from build123d import *

# Parameters (mm, degrees)
SKETCH_1_R      = 27
EXTRUDE_1_DEPTH = 47


with BuildPart() as part:
    # Эскиз1 → Бобышка-Вытянуть1 (new body)
    with BuildSketch(Plane(origin=(0, 0, 0), x_dir=(1, 0, 0), z_dir=(0, 1, 0))):
        with BuildLine():
            ThreePointArc((47, 0), (33.234018716, 33.234018716), (0, 47))
            ThreePointArc((0, 47), (-33.234018716, 33.234018716), (-47, 0))
            ThreePointArc((-47, 0), (-33.234018716, -33.234018716), (0, -47))
            ThreePointArc((0, -47), (33.234018716, -33.234018716), (47, 0))
        make_face()
        Circle(SKETCH_1_R, mode=Mode.SUBTRACT)
        with BuildLine():
            ThreePointArc((-47, 0), (-43.422338028, 17.986121321), (-33.234018716, 33.234018716))
            Line((-33.234018716, 33.234018716), (-56.922095886, 56.922095886))
            ThreePointArc((-56.922095886, 56.922095886), (-57.279535343, 27.533981904), (-47, 0))
        make_face()
        with BuildLine():
            ThreePointArc((-33.234018716, 33.234018716), (-17.986121321, 43.422338028), (0, 47))
            Line((0, 47), (0, 80.5))
            ThreePointArc((0, 80.5), (-21.033282547, 59.972213182), (-33.234018716, 33.234018716))
        make_face()
        with BuildLine():
            Line((33.234018716, 33.234018716), (56.922095886, 56.922095886))
            ThreePointArc((56.922095886, 56.922095886), (27.533981904, 57.279535343), (0, 47))
            ThreePointArc((0, 47), (17.986121321, 43.422338028), (33.234018716, 33.234018716))
        make_face()
        with BuildLine():
            ThreePointArc((80.5, 0), (59.972213182, 21.033282547), (33.234018716, 33.234018716))
            ThreePointArc((33.234018716, 33.234018716), (43.422338028, 17.986121321), (47, 0))
            Line((47, 0), (80.5, 0))
        make_face()
        with BuildLine():
            ThreePointArc((56.922095886, -56.922095886), (57.279535343, -27.533981904), (47, 0))
            ThreePointArc((47, 0), (43.422338028, -17.986121321), (33.234018716, -33.234018716))
            Line((33.234018716, -33.234018716), (56.922095886, -56.922095886))
        make_face()
        with BuildLine():
            ThreePointArc((0, -80.5), (21.033282547, -59.972213182), (33.234018716, -33.234018716))
            ThreePointArc((33.234018716, -33.234018716), (17.986121321, -43.422338028), (0, -47))
            Line((0, -47), (0, -80.5))
        make_face()
        with BuildLine():
            ThreePointArc((-56.922095886, -56.922095886), (-27.533981904, -57.279535343), (0, -47))
            ThreePointArc((0, -47), (-17.986121321, -43.422338028), (-33.234018716, -33.234018716))
            Line((-33.234018716, -33.234018716), (-56.922095886, -56.922095886))
        make_face()
        with BuildLine():
            ThreePointArc((-33.234018716, -33.234018716), (-43.422338028, -17.986121321), (-47, 0))
            Line((-47, 0), (-80.5, 0))
            ThreePointArc((-80.5, 0), (-59.972213182, -21.033282547), (-33.234018716, -33.234018716))
        make_face()
    extrude(amount=EXTRUDE_1_DEPTH)


solid = part.part
Read the model definition and answer for the solid it produces. Units are mm, in the model's axes. A direction names the side the tool comes from. Round coordinates to 2 decimals unless told otherwise and drop trailing zeros. Order: outer loops, then holes, each group sorted by start corner. A loop starts at its lowest first (then second) coordinate and runs counter-clockwise, first axis right, second up.
1) The part is cut by section A-A on z = -9. Write down the section's boundary in (x, y), plus the area to 3 significant figures.
2) The part is cut by section C-C on x = 18. Write down the section's boundary in (y, z).
3) Straight lines are drawn through the part: L1, parallel to X at y = 5, z = 50; L2, parallel to X at y = 21, z = 24; L3, parallel to Z at x = -8.5, y = 44.5. For each, find the intervals that lie inside material, in ascending order.
4) The mould has two halves that part along X. Classify faces 5 (the face through (64, 23, 0)), 6 (the face through (45, 23, -45)), 7 (the face through (-20.8, 23.2, -60.3)): released by +X, released by -X, zero draft, split by the parting line, or undercut.
5) Flat-ended cylindrical pins translate along their axes: pin 1 (6 mm diameter, centred on y = 23, z = -64, fed in from -X); pin 2 (2 mm diameter, centred on x = 2, y = 19.5, fed in from -Z); pin 3 (10 mm diameter, centred on y = 22.5, z = 69.5, fed in from -X). Find the tip coordinate at first contact, or state that the pin passes through.
6) The part is cut by section D-D on z = 50.5. Write down the section's boundary in (x, y), plus the area to 3 significant figures.
7) For faces 1 (the face through (-64, 23, 0)), 2 (the face through (0, 23, -64)), 3 (the face through (-12.3, 47, -24.23)), 4 (the face through (0, 23, 64)), determine the directions among +Z, -Z, +X, -X, +Y, -Y from which every point of the face is accessible in a straight line to the end or side of a thin tool.
8) The part is cut by section B-B on y = 17. Write down the section's boundary in (x, z), plus the area to 3 significant figures.
Resolved:
1. outline: (-51.67, 0) - (-25.46, 0) - (-25.46, 47) - (-51.67, 47) - close; (25.46, 0) - (73.52, 0) - (73.52, 47) - (25.46, 47) - close
1. area: 3,490 mm2
2. outline: (0, -55.01) - (47, -55.01) - (47, -20.12) - (0, -20.12) - close; (0, 20.12) - (47, 20.12) - (47, 64.01) - (0, 64.01) - close
3. L1: x = -50 to -5.45, 0 to 27.01, 50 to 57.99
3. L2: x = -55.43 to -12.37, 12.37 to 56.58
3. L3: z = -73.96 to -25.63, 25.63 to 51.45
4. face 5: zero draft
4. face 6: released by +X
4. face 7: undercut
5. pin 1: stops at x = -20.3
5. pin 2: stops at z = -48.72
5. pin 3: stops at x = 0
6. outline: (-50.5, 0) - (-6.47, 0) - (-6.47, 47) - (-50.5, 47) - close; (0, 0) - (26.76, 0) - (26.76, 47) - (0, 47) - close; (50.5, 0) - (57.93, 0) - (57.93, 47) - (50.5, 47) - close
6. area: 3,680 mm2
7. face 1: -X, +Y, -Y
7. face 2: -Z, +Y, -Y
7. face 3: +Z, -Z, +X, -X, +Y
7. face 4: +Z, +Y, -Y
8. outline: (-80.5, 0) - (-47, 0) arc R80 ccw to (-56.92, -56.92) - (-33.23, -33.23) arc R80 ccw to (0, -80.5) - (0, -47) arc R80 ccw to (56.92, -56.92) - (33.23, -33.23) arc R80 ccw to (80.5, 0) - (47, 0) arc R80 ccw to (56.92, 56.92) - (33.23, 33.23) arc R80 ccw to (0, 80.5) - (0, 47) arc R80 ccw to (-56.92, 56.92) - (-33.23, 33.23) arc R80 ccw to start; hole circle Ø54 at (0, 0)
8. area: 10,100 mm2
